Geometry: final body of the model. Coordinates: model frame, mm. A direction names the side the tool comes from. Coordinates: 2 decimals unless noted, no trailing zeros. Loops run counter-clockwise (first coordinate to the right, second up) from the corner with the lowest first, then second, coordinate; pieces in that order, holes last. Notation, with made-up numbers: M 19,70.25 L 55,70.25 A20 ccw 55,97.25 Z; hole C -31.5,-7.5 d3. An arc over 180 degrees is marked long. Write each question's results on one line, items separated by ' | '. Start each with the question number.
from build123d import *

# Parameters (mm, degrees)
F1_DEPTH = 50.8
F3_DEPTH = 50.8
F4_W     = 25.4
F4_H     = 41.4527870002
F5_DEPTH = 25.4


with BuildPart() as f1:
    # F0 (on Top) → F1 (new body)
    with BuildSketch(Plane.XY):
        Polygon((-12.7, 0), (0, 0), (0, 50.8), (-12.7, 50.8), (-12.7, 37.5397042634), (-25.4, 37.5397042634), (-25.4, 12.1397042634), (-12.7, 12.1397042634), align=None)
    extrude(amount=F1_DEPTH)

    # F2 (on face) → F3 (join)
    with BuildSketch(Plane.XZ):
        Polygon((0, 50.8), (0, 0), (25.4, 0), (25.4, 25.4), align=None)
    extrude(amount=-F3_DEPTH)

    # F4 (on face) → F5 (cut)
    with BuildSketch(Plane.YZ.offset(25.4)):
        with Locations((25.7822034553, 20.7263935001)):
            Rectangle(F4_W, F4_H)
    extrude(amount=-F5_DEPTH, mode=Mode.SUBTRACT)


solid = f1.part
Item 1: Section D-D, the plane x = 1. Return loops of the section in (y, z), plus the area to 3 significant figures.
Item 2: Pull-direction query (Y, two-part tool) for faces 4 (the flat face through (13, 38.482, 20)), 5 (the flat face through (0, 26, 21)), 6 (the flat face through (-25.4, 25, 25)), 7 (the flat face through (-19, 12.14, 25)); classes: released by +Y, released by -Y, zero draft, split by the parting line, or undercut.
Item 3: Set-up query: faces 1 (the flat face through (5, 26, 41.453)), 2 (the flat face through (-19, 37.54, 25)), 3 (the flat face through (-12.7, 6, 25)). Return all of +Z, -Z, +X, -X, +Y, -Y with unobstructed straight access to the full face (end or side cutting, diameter ignored); none if empty.
Item 4: Contact query for flat-ended pins moving along their axis: P1, Ø6.5, axis at x = -18, z = 16.5, coming from the +Y side; P2, Ø12, axis at y = 44, z = 21.5, coming from the -X side; P3, Ø6.5, axis at x = -18, z = 38, coming from the -Y side. Output: stop coordinate, or through.
Item 5: Section C-C, the plane y = 3.5. Return loops of the section in (x, z).
Item 6: Section A-A, the plane x = 20. Return loops of the section in (y, z).
Item 7: Ray query, L1, parallel to Y at x = 1.5, z = 41; L2, parallel to X at y = 20, z = 10; L3, parallel to X at y = 11.5, z = 12. Return the intervals inside material, ascending. Write a range as [from, to].
Item 8: Section B-B, the plane z = 44. Return loops of the section in (x, y), plus the area to 3 significant figures.
Solutions:
1) outline: M 0,0 L 13.08,0 L 13.08,41.45 L 38.48,41.45 L 38.48,0 L 50.8,0 L 50.8,49.8 L 0,49.8 Z | area: 1,480 mm²
2) face 4: undercut | face 5: undercut | face 6: zero draft | face 7: released by -Y
3) face 1: -Z, +X | face 2: +Z, -Z, -X, +Y | face 3: +Z, -Z, -X, -Y
4) P1: stops at y = 37.54 | P2: stops at x = -12.7 | P3: stops at y = 12.14
5) outline: M -12.7,0 L 25.4,0 L 25.4,25.4 L 0,50.8 L -12.7,50.8 Z
6) outline: M 0,0 L 13.08,0 L 13.08,30.8 L 0,30.8 Z; M 38.48,0 L 50.8,0 L 50.8,30.8 L 38.48,30.8 Z
7) L1: y = [0, 13.08], [38.48, 50.8] | L2: x = [-25.4, 0] | L3: x = [-12.7, 25.4]
8) outline: M -25.4,12.14 L -12.7,12.14 L -12.7,0 L 6.8,0 L 6.8,50.8 L -12.7,50.8 L -12.7,37.54 L -25.4,37.54 Z | area: 1,310 mm²
